Check sheet for the modelled part. Datum: model origin and axes. Units: mm. A direction names the side the tool comes from. Give positions to 0.01 mm unless a question says otherwise; leave off trailing zeros. Loops run counter-clockwise (first coordinate to the right, second up) from the corner with the lowest first, then second, coordinate; pieces in that order, holes last. Notation, with made-up numbers: (-9.5, 15) - (-1.5, 15) arc R3 ccw to (-1.5, 20) - close; hole circle Ø7 at (64, 47.25). An arc over 180 degrees is marked (long way). Use CSV: the item, a comma, the result in double quotes.
from build123d import *

# Parameters (mm, degrees)
SKETCH2_W             = 47
SKETCH2_H             = 16.65
BOSS_EXTRUDE1_DEPTH   = 3.175
FILLET1_R             = 3.175
FILLET2_R             = 12.7
F_2_CLEARANCE_HOLE1_D = 2.7051
F_2_CLEARANCE_HOLE2_D = 2.7051


with BuildPart() as part:
    # Sketch2 → Boss-Extrude1 (new body)
    with BuildSketch(Plane.XY):
        with BuildLine():
            Line((58.628990163, 28.900566469), (52.80618907, 26.175))
            Line((52.80618907, 26.175), (7.206212285, 26.175))
            Line((7.206212285, 26.175), (1.299208473, 28.885670965))
            ThreePointArc((1.299208473, 28.885670965), (-1.739097882, 28.672544378), (-3.2, 26))
            Line((-3.2, 26), (-3.175, 0))
            ThreePointArc((-3.175, 0), (-2.24506403, -2.24506403), (0, -3.175))
            Line((0, -3.175), (60.025, -3.175))
            ThreePointArc((60.025, -3.175), (62.272219886, -2.242906103), (63.199994139, 0.006100608))
            Line((63.199994139, 0.006100608), (63.15, 26.025))
            ThreePointArc((63.15, 26.025), (61.678972384, 28.704011593), (58.628990163, 28.900566469))
        make_face()
        with Locations((30.0125, 11.5)):
            Rectangle(SKETCH2_W, SKETCH2_H, mode=Mode.SUBTRACT)
    extrude(amount=BOSS_EXTRUDE1_DEPTH)

    # Fillet1
    fillet1_edges = [part.edges().sort_by_distance(p)[0] for p in [
        (6.5125, 3.175, 1.5875),
        (53.5125, 3.175, 1.5875),
        (53.5125, 19.825, 1.5875),
        (6.5125, 19.825, 1.5875),
    ]]
    fillet(fillet1_edges, radius=FILLET1_R)

    # Fillet2
    fillet2_edges = [part.edges().sort_by_distance(p)[0] for p in [
        (7.206212285, 26.175, 1.5875),
        (52.80618907, 26.175, 1.5875),
    ]]
    fillet(fillet2_edges, radius=FILLET2_R)

    # #2 Clearance Hole1 (through all)
    with Locations(Plane.XY.offset(3.175)):
        with Locations((6.5125, 23), (53.5125, 23), (53.5125, 0), (6.5125, 0)):
            Hole(F_2_CLEARANCE_HOLE1_D / 2)

    # #2 Clearance Hole2 (through all)
    with Locations(Plane.XY.offset(3.175)):
        with Locations((-0.025, 26), (0, 0), (60.025, 0), (59.975, 26.025)):
            Hole(F_2_CLEARANCE_HOLE2_D / 2)


solid = part.part
1. Sectioned sample at B-B, the plane z = 1.55. State how many separate pieces and enclosed holes the cut face has, and give its area (3 significant figures).
Completed:
separate pieces,"1"
enclosed holes,"9"
area,"1,160 mm²"
2. Sectioned sample at C-C, the plane y = 23. Record the boundary of the cut face in (x, z) (3 decimals), and give its area (3 significant figures).
Completed:
outline,"(-3.197, 0) - (5.16, 0) - (5.16, 3.175) - (-3.197, 3.175) - close; (7.865, 0) - (52.16, 0) - (52.16, 3.175) - (7.865, 3.175) - close; (54.865, 0) - (63.156, 0) - (63.156, 3.175) - (54.865, 3.175) - close"
area,"193 mm²"
3. Scan lines: line 1 along Y through (x, z) = (0, 2.1) (3 decimals); line 2 along X through (y, z) = (0.5, 2.7); line 3 along X through (y, z) = (7.5, 2.4). Record each from-to range of solid material in increasing order.
Completed:
line 1,"y = -3.175 to -1.353, 1.353 to 24.648, 27.352 to 29.175"
line 2,"x = -3.18 to -1.26, 1.26 to 5.26, 7.77 to 52.26, 54.77 to 58.77, 61.28 to 63.2"
line 3,"x = -3.18 to 6.51, 53.51 to 63.19"
4. Sectioned sample at A-A, the plane x = 43. Record the boundary of the cut face in (y, z) (3 decimals).
Completed:
outline,"(-3.175, 0) - (3.175, 0) - (3.175, 3.175) - (-3.175, 3.175) - close; (19.825, 0) - (26.175, 0) - (26.175, 3.175) - (19.825, 3.175) - close"
5. Release check for a two-part mould opening along Y. For faces 3 (the face through (30, 20, 3.175)), 4 (the face through (7.31, 26.46, 1.61)), 5 (the face through (-0.65, 24.8, 1.57)) record: released by +Y, released by -Y, zero draft, split by the parting line, or undercut.
Completed:
face 3,"zero draft"
face 4,"released by +Y"
face 5,"undercut"
6. Sectioned sample at D-D, the plane y = 8. Record the boundary of the cut face in (x, z) (1 decimal), and give its area (3 significant figures).
Completed:
outline,"(-3.2, 0) - (6.5, 0) - (6.5, 3.2) - (-3.2, 3.2) - close; (53.5, 0) - (63.2, 0) - (63.2, 3.2) - (53.5, 3.2) - close"
area,"61.5 mm²"
7. Set-up check for faces 1 (the face through (52.56, 4.08, 1.61)), 2 (the face through (30, 26.175, 2)): record each of +Z, -Z, +X, -X, +Y, -Y from which the full face is reachable in a straight line by a thin tool's end or side.
Completed:
face 1,"+Z, -Z"
face 2,"+Z, -Z, +Y"
8. Go/stop test with flat-tipped pins: pin 1 Ø1 at (y, z) = (10, 2.5) entering from +X; pin 2 Ø2.5 at (x, y) = (60.025, 0) entering from +Z. Record where each tip stops, or that it passes through.
Completed:
pin 1,"stops at x = 63.18"
pin 2,"passes through"
